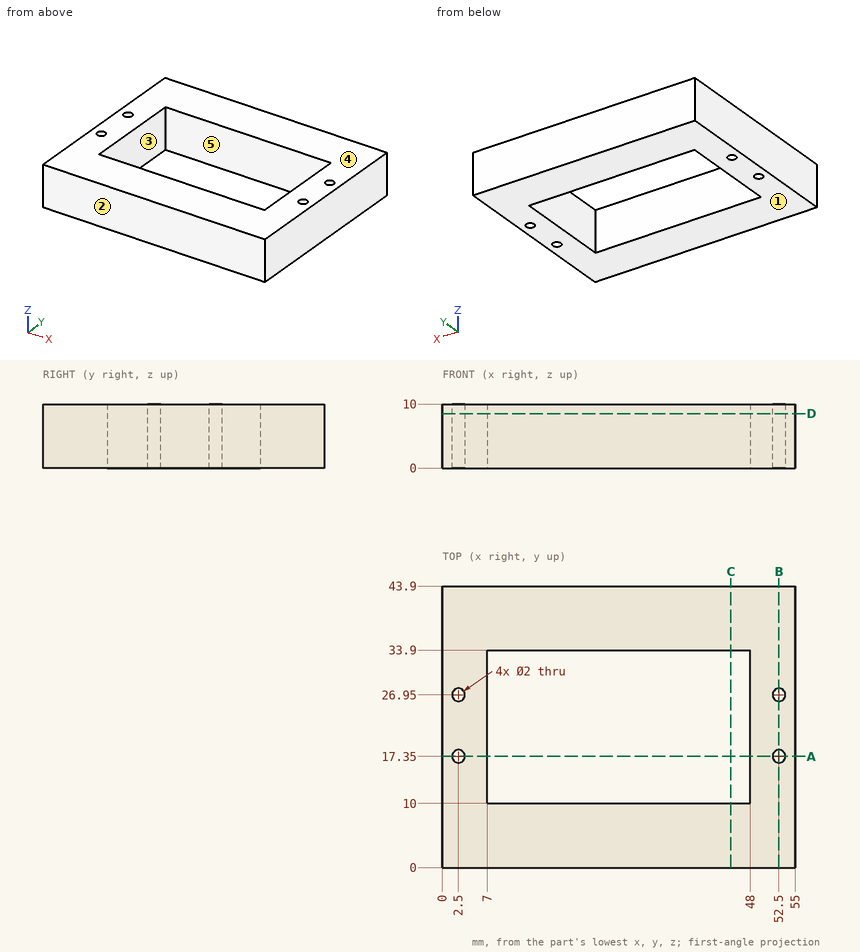
Answer from the drawing. Dimensions are ordinates in mm from the lowest x, y and z of the part. A direction names the side the tool comes from. Round coordinates to 2 decimals unless told otherwise and drop trailing zeros. Loops run counter-clockwise (first coordinate to the right, second up) from the corner with the lowest first, then second, coordinate; pieces in that order, holes last. Notation, with made-up numbers: (25.25, 67) - (70.25, 67) arc R33 ccw to (70.25, 103) - close; hole circle Ø7 at (68.5, -19.5). An arc over 180 degrees is marked (long way). Return JSON: item names as keys, results as strings. Group by question number.
1. The mould has two halves that part along Y. Classify the marked faces 1, 2 and 3: pulls with the +Y half, pulls with the -Y half, needs draft (parallel to the pull), parting line crosses it, or undercut.
2. The part is cut by section B-B on x = 52.5. Determine the outline of the cut face in (y, z).
3. Consider probe 1 along X at (y, z) = (17.35, 2.5); probe 2 along Y at (x, z) = (52.5, 2.75); probe 3 along Y at (x, z) = (27.5, 1.5). Determine where each line is inside the solid, lowest interval first.
4. Which of the six approach directions +Z, -Z, +X, -X, +Y, -Y give full straight-line access (tool end or side, diameter ignored) to the marked faces 4 and 5?
5. The part is cut by section A-A on y = 17.35. Determine the outline of the cut face in (x, z).
6. This flat-tipped pin is pushed along its axis until it touches: P1, Ø1.8, axis at x = 2.5, y = 26.95, coming from the +Z side. Where does it stop, or does it pass through?
7. The part is cut by section C-C on x = 45. Determine the outline of the cut face in (y, z).
8. The part is cut by section D-D on z = 8.5. Determine the outline of the cut face in (x, y), then the cut area to 3 significant figures.
Resolved:
{
 "1": {"face 1": "needs draft", "face 2": "pulls with the -Y half", "face 3": "undercut"},
 "2": {"outline": "(0, 0) - (16.35, 0) - (16.35, 10) - (0, 10) - close; (18.35, 0) - (25.95, 0) - (25.95, 10) - (18.35, 10) - close; (27.95, 0) - (43.9, 0) - (43.9, 10) - (27.95, 10) - close"},
 "3": {"probe 1": "x = 0 to 1.5, 3.5 to 7, 48 to 51.5, 53.5 to 55", "probe 2": "y = 0 to 16.35, 18.35 to 25.95, 27.95 to 43.9", "probe 3": "y = 0 to 10, 33.9 to 43.9"},
 "4": {"face 4": "+Z, +X, -X, +Y, -Y", "face 5": "+Z, -Z"},
 "5": {"outline": "(0, 0) - (1.5, 0) - (1.5, 10) - (0, 10) - close; (3.5, 0) - (7, 0) - (7, 10) - (3.5, 10) - close; (48, 0) - (51.5, 0) - (51.5, 10) - (48, 10) - close; (53.5, 0) - (55, 0) - (55, 10) - (53.5, 10) - close"},
 "6": {"P1": "passes through"},
 "7": {"outline": "(0, 0) - (10, 0) - (10, 10) - (0, 10) - close; (33.9, 0) - (43.9, 0) - (43.9, 10) - (33.9, 10) - close"},
 "8": {"outline": "(0, 0) - (55, 0) - (55, 43.9) - (0, 43.9) - close; hole circle Ø2 at (2.5, 17.35); hole circle Ø2 at (2.5, 26.95); hole (7, 10) - (48, 10) - (48, 33.9) - (7, 33.9) - close; hole circle Ø2 at (52.5, 17.35); hole circle Ø2 at (52.5, 26.95)", "area": "1,420 mm²"}
}
